from build123d import *

# Parameters (mm, degrees)
SKETCH_1_R      = 15
EXTRUDE_1_DEPTH = 15
SKETCH_2_R      = 24
EXTRUDE_2_DEPTH = 280
SCALE_1_SCALE   = 0.6


with BuildPart() as part:
    # 草图1 → 凸台-拉伸1 (new body)
    with BuildSketch(Plane.XY):
        with BuildLine():
            Line((0, 25), (60, 25))
            Line((60, 25), (60, -25))
            Line((60, -25), (0, -25))
            ThreePointArc((0, -25), (-25, 0), (0, 25))
        make_face()
        Circle(SKETCH_1_R, mode=Mode.SUBTRACT)
    extrude(amount=EXTRUDE_1_DEPTH)

    # 草图2 → 凸台-拉伸2 (add)
    with BuildSketch(Plane(origin=(60, 0, 0), x_dir=(0, 0, -1), z_dir=(1, 0, 0))):
        with Locations(Location((-7.5, 0, 0), (0, 0, 108.209956864))):
            Circle(SKETCH_2_R)
    extrude(amount=EXTRUDE_2_DEPTH)


with BuildPart() as part_1:
    # 缩放比例1: scaled about (0, 0, 0)
    add(part.part.scale(SCALE_1_SCALE))


solid = part_1.part
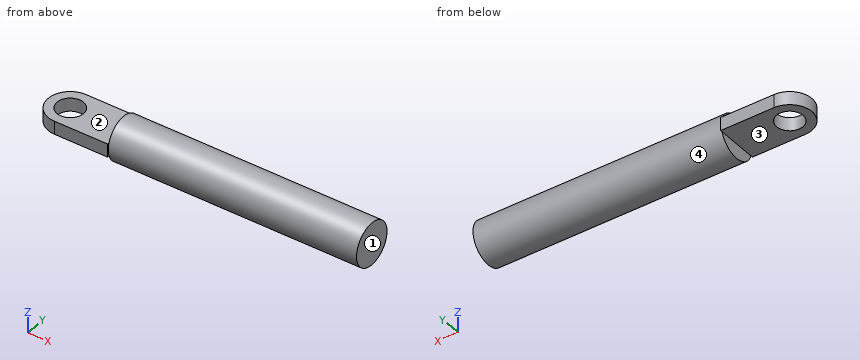
Can you work these out from the model? Positions are in its coordinate system, mm. Face numbers are marked on the shaded views. A direction names the side the tool comes from. Give positions to 0.01 mm unless a question says otherwise; leave off trailing zeros. Write each loop counter-clockwise with the first axis right and the second up, starting at its lowest first coordinate (ties: lowest second). Pieces come first, ordered by that corner, then holes. Notation, with made-up numbers: (34.25, 11.5) -> (88.25, 11.5) arc R7 cw to (88.25, 15.5) -> close; hole circle Ø6 at (-36.75, 85). An arc over 180 degrees is marked (long way). Answer as a JSON object with one key per item and string values. Group by question number.
Item 1: I'm going to push flat-ended pins straight in: P1, Ø15, axis at x = 0, y = -2.5, coming from the -Z side; P2, Ø11, axis at y = 4.5, z = 15, coming from the -X side; P3, Ø11, axis at y = -3, z = -5, coming from the -X side; P4, Ø1.1, axis at y = 14.5, z = 6, coming from the +X side. Where does each tip first touch, or does it pass through?
Item 2: Suppose I cut it at A-A (z = 4.5). Please give me the cut outline in (x, y), plus the area to 3 significant figures.
Item 3: Suppose I cut it at D-D (y = 11.5). Please give me the cut outline in (x, z), plus the area to 3 significant figures.
Item 4: Suppose I cut it at B-B (y = 0). Please give me the cut outline in (x, z).
Item 5: Suppose I cut it at C-C (x = 173). Please give me the cut outline in (y, z).
Item 6: For the marked faces 1, 2, 3 and 4, which set-ups out of +Z, -Z, +X, -X, +Y, -Y let a thin tool reach every point of the face, with its end or its side?
Item 7: Please list where these lines run through material, in increasing order: line 1 (Y direction, x = 0, z = 2); line 2 (X direction, y = 9.75, z = 12); line 3 (X direction, y = -8, z = 1.75). Write a range as [from, to].
Findings:
{
 "1": {"P1": "stops at z = 0", "P2": "stops at x = 36", "P3": "stops at x = -14.98", "P4": "stops at x = 204"},
 "2": {"outline": "(0, -15) -> (36, -15) -> (36, -14.4) -> (204, -14.4) -> (204, 14.4) -> (36, 14.4) -> (36, 15) -> (0, 15) arc R15 ccw to start; hole circle Ø18 at (0, 0)", "area": "6,020 mm²"},
 "3": {"outline": "(-9.63, 0) -> (36, 0) -> (36, -4.17) -> (204, -4.17) -> (204, 13.17) -> (36, 13.17) -> (36, 9) -> (-9.63, 9) -> close", "area": "3,320 mm²"},
 "4": {"outline": "(-15, 0) -> (-9, 0) -> (-9, 9) -> (-15, 9) -> close; (9, 0) -> (36, 0) -> (36, -9.9) -> (204, -9.9) -> (204, 18.9) -> (36, 18.9) -> (36, 9) -> (9, 9) -> close"},
 "5": {"outline": "circle Ø28.8 at (0, 4.5)"},
 "6": {"face 1": "+Z, -Z, +X, +Y, -Y", "face 2": "+Z, -X, +Y, -Y", "face 3": "-Z, -X, +Y, -Y", "face 4": "+X"},
 "7": {"line 1": "y = [-15, -9], [9, 15]", "line 2": "x = [36, 204]", "line 3": "x = [-12.69, -4.12], [4.12, 204]"}
}
